```python
from build123d import *

# Parameters (mm, degrees)
SKETCH1_W           = 126
SKETCH1_H           = 130
SKETCH1_R           = 1.5
BOSS_EXTRUDE1_DEPTH = 10
SKETCH3_W           = 126
SKETCH3_H           = 5
BOSS_EXTRUDE2_DEPTH = 82
BOSS_EXTRUDE4_DEPTH = 126
SKETCH5_R           = 1.5
CUT_EXTRUDE1_DEPTH  = 3
SKETCH6_R           = 1.5
CUT_EXTRUDE2_DEPTH  = 2
CHAMFER1_SIZE       = 3


with BuildPart() as part:
    # Sketch1 → Boss-Extrude1 (new body)
    with BuildSketch(Plane(origin=(0, 0, 0), x_dir=(1, 0, 0), z_dir=(0, 1, 0))):
        with Locations((63, -65)):
            Rectangle(SKETCH1_W, SKETCH1_H)
        with Locations(Location((38, -40, 0), (0, 0, 270))):
            Circle(SKETCH1_R, mode=Mode.SUBTRACT)
        with Locations(Location((88, -40, 0), (0, 0, 270))):
            Circle(SKETCH1_R, mode=Mode.SUBTRACT)
        with Locations(Location((88, -90, 0), (0, 0, 270))):
            Circle(SKETCH1_R, mode=Mode.SUBTRACT)
        with Locations(Location((38, -90, 0), (0, 0, 270))):
            Circle(SKETCH1_R, mode=Mode.SUBTRACT)
    extrude(amount=BOSS_EXTRUDE1_DEPTH)

    # Sketch3 → Boss-Extrude2 (add)
    with BuildSketch(Plane.XZ):
        with Locations((63, 127.5)):
            Rectangle(SKETCH3_W, SKETCH3_H)
        with Locations((63, 2.5)):
            Rectangle(SKETCH3_W, SKETCH3_H)
    extrude(amount=BOSS_EXTRUDE2_DEPTH)

    # Sketch4 → Boss-Extrude4 (add)
    with BuildSketch(Plane(origin=(126, 0, 0), x_dir=(0, 0, -1), z_dir=(1, 0, 0))):
        Polygon((-125, -74), (-125, -82), (-81, -82), (-81, -76), (-65, -76), (-65, -74), align=None)
        Polygon((-81, -76), (-81, -82), (-79, -82), (-79, -78), (-65, -78), (-65, -76), align=None)
        Polygon((-79, -82), (-81, -82), (-81, -101), (-49, -101), (-49, -82), (-51, -82), (-51, -98), (-79, -98), align=None)
        Polygon((-49, -76), (-65, -76), (-65, -78), (-51, -78), (-51, -82), (-49, -82), align=None)
        Polygon((-5, -74), (-65, -74), (-65, -76), (-49, -76), (-49, -82), (-5, -82), align=None)
    extrude(amount=-BOSS_EXTRUDE4_DEPTH)

    # Sketch5 → Cut-Extrude1 (cut)
    with BuildSketch(Plane.XZ.offset(101)):
        with Locations(Location((25, 65, 0), (0, 0, 270))):
            Circle(SKETCH5_R)
        with Locations(Location((63, 65, 0), (0, 0, 270))):
            Circle(SKETCH5_R)
        with Locations(Location((101, 65, 0), (0, 0, 270))):
            Circle(SKETCH5_R)
    extrude(amount=-CUT_EXTRUDE1_DEPTH, mode=Mode.SUBTRACT)

    # Sketch6 → Cut-Extrude2 (cut)
    with BuildSketch(Plane.XY.offset(81)):
        with Locations((106, -91)):
            Circle(SKETCH6_R)
        with Locations((63, -91)):
            Circle(SKETCH6_R)
        with Locations((20, -91)):
            Circle(SKETCH6_R)
    extrude(amount=-CUT_EXTRUDE2_DEPTH, mode=Mode.SUBTRACT)

    # Chamfer1
    chamfer1_edges = [part.edges().sort_by_distance(p)[0] for p in [
        (63, 10, 0),
        (63, 0, 125),
        (63, -82, 130),
        (63, 0, 5),
        (63, -82, 0),
        (63, -78, 51),
        (63, -78, 79),
        (63, -98, 79),
        (63, -82, 49),
        (63, -101, 49),
        (63, -101, 81),
        (63, -82, 81),
        (63, -74, 125),
        (63, -74, 5),
        (63, -98, 51),
        (63, 10, 130),
    ]]
    chamfer(chamfer1_edges, length=CHAMFER1_SIZE)


solid = part.part
```
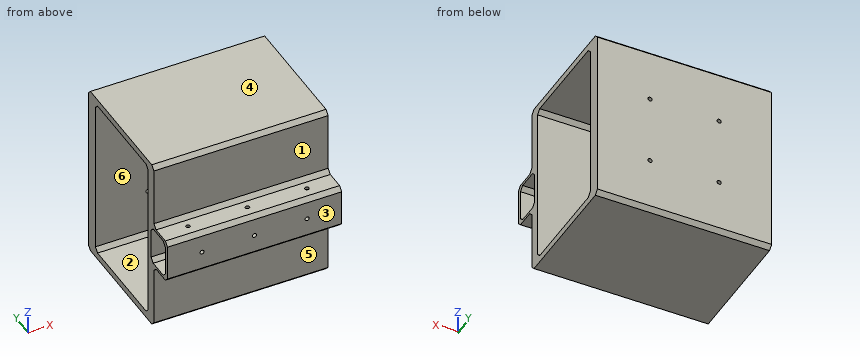
Design review of the part built by this model. Coordinates are the model's own, in mm. Face numbers are marked on the shaded views. A direction names the side the tool comes from. Give positions to 0.01 mm unless a question says otherwise; leave off trailing zeros. Order: outer loops, then holes, each group sorted by start corner. A loop starts at its lowest first (then second) coordinate and runs counter-clockwise, first axis right, second up. Notation, with made-up numbers: (18.5, 57) - (60.5, 57) arc R11 ccw to (60.5, 63) - close; hole circle Ø6 at (60.5, 89.25). An arc over 180 degrees is marked (long way). Use a Markdown table: item, result. Add a question column.
(1) Clearance check with flat-ended pins moving along their axes: P1, Ø3, axis at y = -88.5, z = 83.5, coming from the +X side; P2, Ø10.5, axis at x = 72.5, y = -91, coming from the -Z side; P3, Ø2.5, axis at x = 38, z = 90, coming from the -Y side; P4, Ø1.8, axis at x = 25, z = 65, coming from the -Y side. State where each tip first meets the part, or that it passes through.
(2) Wall thickness on probe 1 along Y at (x, z) = (45, 74.5); probe 2 along X at (y, z) = (-99, 65); probe 3 along X at (y, z) = (5.5, 40): over which ranges is each line inside the solid? List them lowest first. Write a range as [from, to].
(3) Mouldability with a two-part tool opening along Z and no side actions: class the marked faces 4, 5 and 6 as +Z half, -Z half, draft (parallel to the pull), parting line (faces both ways), or undercut.
(4) Add section A-A on x = 80.5. Give the number of separate pieces and of enclosed holes in the cut face, then the cut area to 3 significant figures.
(5) Add section B-B on y = -53. Give the boundary of the cut face in (x, z).
(6) Machinability: for the marked faces 1, 2 and 3, which of the approach directions +Z, -Z, +X, -X, +Y, -Y give a long, thin tool a straight path to every point of the face, cutting with its end or side? Answer none if there is none.
Report:
| question | item | result |
|---|---|---|
| 1 | P1 | passes through |
| 1 | P2 | stops at z = 49 |
| 1 | P3 | stops at y = -82 |
| 1 | P4 | stops at y = -78 |
| 2 | probe 1 | y = [-101, -98], [-78, -74], [0, 10] |
| 2 | probe 2 | x = [0, 23.5], [26.5, 61.5], [64.5, 99.5], [102.5, 126] |
| 2 | probe 3 | x = [0, 36.5], [39.5, 86.5], [89.5, 126] |
| 3 | face 4 | +Z half |
| 3 | face 5 | draft |
| 3 | face 6 | undercut |
| 4 | separate pieces | 1 |
| 4 | enclosed holes | 2 |
| 4 | area | 3,150 mm² |
| 5 | outline | (0, 0) - (126, 0) - (126, 5) - (0, 5) - close; (0, 125) - (126, 125) - (126, 130) - (0, 130) - close |
| 6 | face 1 | +Z, +X, -X, -Y |
| 6 | face 2 | +X, -X |
| 6 | face 3 | +Z, -Z, +X, -X, -Y |
